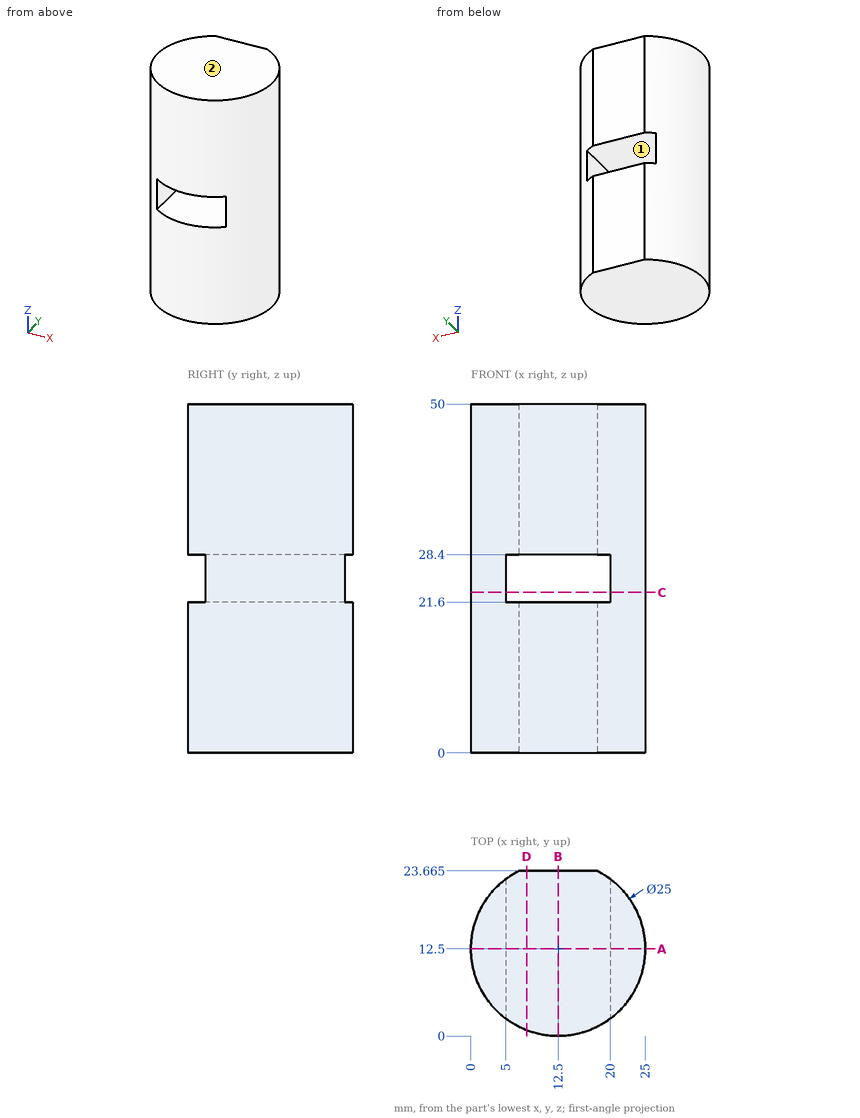
Print and shaded views of the part. All mm, measured from the part's lowest x, y and z. A direction names the side the tool comes from. Coordinates: 2 decimals unless noted, no trailing zeros. Order: outer loops, then holes, each group sorted by start corner. A loop starts at its lowest first (then second) coordinate and runs counter-clockwise, first axis right, second up. Notation, with made-up numbers: M 17,33 L 24,33 A12 cw 24,42 Z; hole C 39,50 d9. An arc over 180 degrees is marked long. One line per question, with ' | ' between items. Start each with the question number.
Q1. Saw through at A-A (y = 12.5). List the corners of the cut face in (x, z), then the cut area to 3 significant figures.
Q2. Saw through at B-B (x = 12.5). List the corners of the cut face in (y, z) (1 decimal).
Q3. Saw through at D-D (x = 8). List the corners of the cut face in (y, z) (1 decimal).
Q4. Flat gauge pins, fed straight in: pin 1 Ø2 at (y, z) = (20.5, 25) entering from -X (1 decimal); pin 2 Ø12 at (y, z) = (10, 30.5) entering from +X; pin 3 Ø12 at (x, z) = (21, 30) entering from -Y; pin 4 Ø1 at (x, z) = (17, 21) entering from -Y. Where does each tip first touch, or does it go through?
Q5. 3-axis set-ups, long thin cutter, end or side, ignore diameter. For the marked faces 1 and 2: which of +Z, -Z, +X, -X, +Y, -Y reach the whole face in a straight line?
Q6. Probe L1, parallel to Z at x = 9.25, y = 20.25; L2, parallel to X at y = 11.5, z = 27; L3, parallel to X at y = 3.5, z = 28 (1 decimal). List the from-to ranges inside material, lowest first. Write a range as from..to.
Q7. Saw through at C-C (z = 23). List the corners of the cut face in (x, y), then the cut area to 3 significant figures.
Check values:
1) outline: M 0,0 L 25,0 L 25,50 L 0,50 Z; hole M 5,21.6 L 20,21.6 L 20,28.4 L 5,28.4 Z | area: 1,150 mm2
2) outline: M 0,0 L 23.7,0 L 23.7,21.6 L 0,21.6 Z; M 0,28.4 L 23.7,28.4 L 23.7,50 L 0,50 Z
3) outline: M 0.8,0 L 23.7,0 L 23.7,21.6 L 0.8,21.6 Z; M 0.8,28.4 L 23.7,28.4 L 23.7,50 L 0.8,50 Z
4) pin 1: stops at x = 2.1 | pin 2: stops at x = 25 | pin 3: stops at y = 0.25 | pin 4: stops at y = 0.66
5) face 1: +Y, -Y | face 2: +Z, +X, -X, +Y, -Y
6) L1: z = 0..21.6, 28.4..50 | L2: x = 0.04..5, 20..24.96 | L3: x = 3.8..5, 20..21.2
7) outline: M 5,2.5 L 5,22.5 A12.5 ccw Z; M 20,2.5 A12.5 ccw 20,22.5 Z | area: 140 mm2
